Build history of the part. All positions in model axes, mm. Give positions to 0.01 mm unless a question says otherwise; leave off trailing zeros. Loops run counter-clockwise (first coordinate to the right, second up) from the corner with the lowest first, then second, coordinate; pieces in that order, holes last.
1) Band-saw the part on A-A on y = 7.75. List the corners of the cut face in (x, z), then the cut area to 3 significant figures.
2) Wall check: line 1 (Z direction, x = 1.55, y = -12.5); line 2 (Y direction, x = 2.4, z = -22); line 3 (Z direction, x = 2.8, y = -0.25). Give the ranges that are in metal, low to high.
3) Flat gauge pins, fed straight in: P1, Ø1.5, axis at x = 2, y = -13.5, coming from the -Z side; P2, Ø2, axis at y = -2.5, z = -12, coming from the -X side; P3, Ø1.5, axis at x = 2, z = -23.5, coming from the -Y side; P4, Ø1.5, axis at x = 2, y = -14, coming from the +Z side. Where does each tip first touch, or does it go through?
4) Band-saw the part on C-C on y = 0.5. List the corners of the cut face in (x, z), then the cut area to 3 significant figures.
5) Band-saw the part on D-D on z = 13. List the corners of the cut face in (x, y).
6) Band-saw the part on B-B on x = 1.2. List the corners of the cut face in (y, z), then the cut area to 3 significant figures.
```python
from build123d import *

# Parameters (mm, degrees)
BOSS_EXTRUDE1_DEPTH = 3
FILLET1_R           = 5
SKETCH3_W           = 3
SKETCH3_H           = 5
BOSS_EXTRUDE2_DEPTH = 3


with BuildPart() as part:
    # Sketch1 → Boss-Extrude1 (new body)
    with BuildSketch(Plane(origin=(0, 0, 0), x_dir=(0, 0, -1), z_dir=(1, 0, 0))):
        with BuildLine():
            Line((-14, 11.75), (-30, 11.75))
            Line((-30, 11.75), (-30, -11.75))
            Line((-30, -11.75), (30, -11.75))
            Line((30, -11.75), (30, 11.75))
            Line((30, 11.75), (14, 11.75))
            ThreePointArc((14, 11.75), (0, -2.25), (-14, 11.75))
        make_face()
    extrude(amount=BOSS_EXTRUDE1_DEPTH)

    # Fillet1
    fillet1_edges = [part.edges().sort_by_distance(p)[0] for p in [
        (1.5, 11.75, 30),
        (1.5, 11.75, -30),
    ]]
    fillet(fillet1_edges, radius=FILLET1_R)

    # Sketch3 → Boss-Extrude2 (add)
    with BuildSketch(Plane.XZ.offset(11.75)):
        with Locations((1.5, 17.5)):
            Rectangle(SKETCH3_W, SKETCH3_H)
    boss_extrude2 = extrude(amount=BOSS_EXTRUDE2_DEPTH)

    # Mirror3: Boss-Extrude2 across plane
    add(boss_extrude2.mirror(Plane.XY))


solid = part.part
```
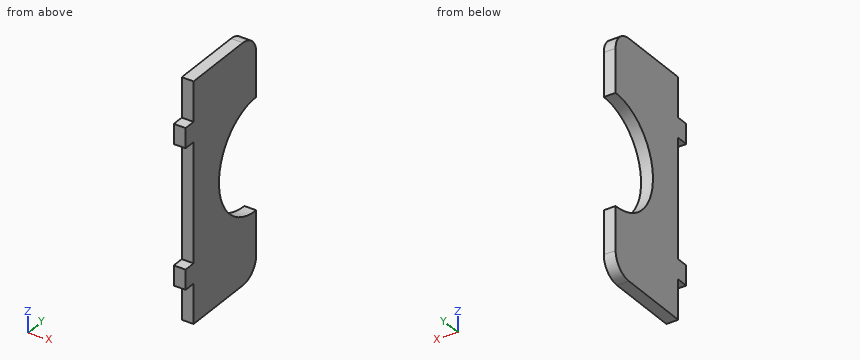
Findings below:
1. outline: (0, -29.9) - (3, -29.9) - (3, -13.42) - (0, -13.42) - close; (0, 13.42) - (3, 13.42) - (3, 29.9) - (0, 29.9) - close
1. area: 98.9 mm2
2. line 1: z = -20 to -15, 15 to 20
2. line 2: y = -11.75 to 11.75
2. line 3: z = -30 to -7.21, 7.21 to 30
3. P1: stops at z = -20
3. P2: stops at x = 0
3. P3: stops at y = -11.75
3. P4: stops at z = 20
4. outline: (0, -30) - (3, -30) - (3, -8.33) - (0, -8.33) - close; (0, 8.33) - (3, 8.33) - (3, 30) - (0, 30) - close
4. area: 130 mm2
5. outline: (0, -11.75) - (3, -11.75) - (3, 6.55) - (0, 6.55) - close
6. outline: (-14.75, -20) - (-11.75, -20) - (-11.75, -30) - (6.75, -30) arc R5 ccw to (11.75, -25) - (11.75, -14) arc R14 cw to (11.75, 14) - (11.75, 25) arc R5 ccw to (6.75, 30) - (-11.75, 30) - (-11.75, 20) - (-14.75, 20) - (-14.75, 15) - (-11.75, 15) - (-11.75, -15) - (-14.75, -15) - close
6. area: 1,120 mm2
